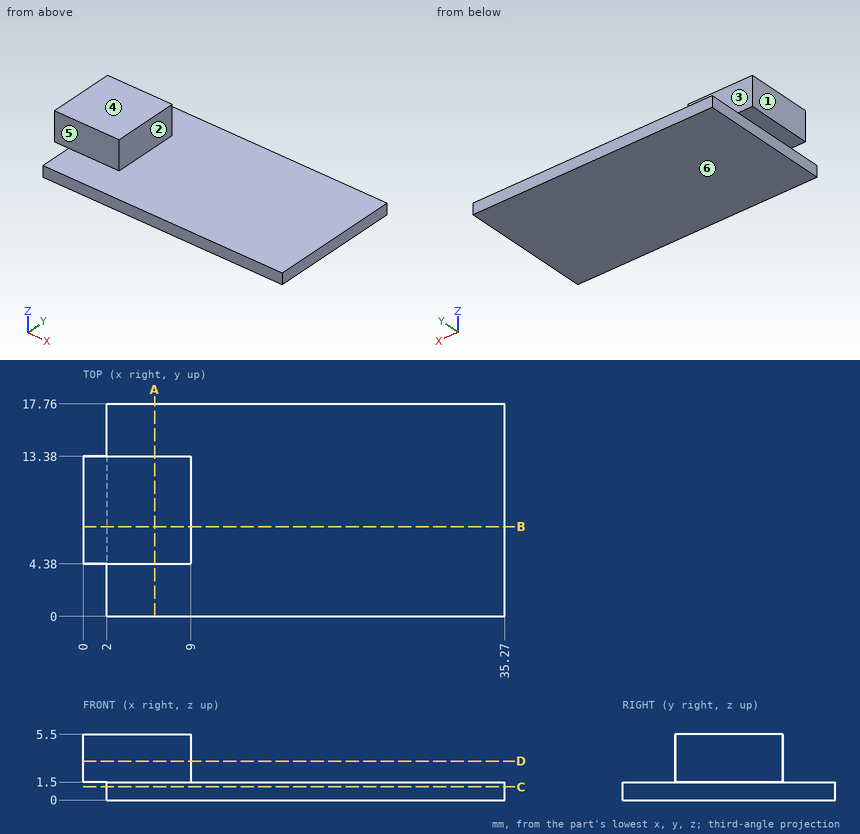
The figure shows three views and two pictorial views of one solid part (mm, origin at its lowest corner). Answer the questions. A direction names the side the tool comes from. Give positions to 0.01 mm unless a question says otherwise; leave off trailing zeros. Write each loop counter-clockwise with the first axis right and the second up, starting at its lowest first coordinate (ties: lowest second). Pieces come first, ordered by that corner, then holes. Notation, with made-up numbers: (32.25, 88.5) -> (56.25, 88.5) arc R34 ccw to (56.25, 118.5) -> close; hole circle Ø4 at (-30.75, 62). An arc over 180 degrees is marked (long way). Write each question's results on one line, items separated by ' | '.
1. Find section B-B on y = 7.5. Determine the outline of the cut face in (x, z).
Data:
outline: (0, 1.5) -> (2, 1.5) -> (2, 0) -> (35.27, 0) -> (35.27, 1.5) -> (9, 1.5) -> (9, 5.5) -> (0, 5.5) -> close
2. Find section C-C on z = 1.1. Determine the outline of the cut face in (x, y), and give its area (3 significant figures).
Data:
outline: (2, 0) -> (35.27, 0) -> (35.27, 17.76) -> (2, 17.76) -> close | area: 591 mm^2
3. Find section D-D on z = 3.25. Determine the outline of the cut face in (x, y), and give its area (3 significant figures).
Data:
outline: (0, 4.38) -> (9, 4.38) -> (9, 13.38) -> (0, 13.38) -> close | area: 81.0 mm^2
4. Each of these flat-tipped pins is pushed along its axis until it touches: pin 1 Ø3 at (x, y) = (27, 14.5) entering from +Z; pin 2 Ø3 at (y, z) = (10, 3.5) entering from +X; pin 3 Ø1.2 at (x, z) = (3.5, 4.5) entering from -Y. Where does it stop, or does it pass through?
Data:
pin 1: z = 1.5 | pin 2: x = 9 | pin 3: y = 4.38
5. A tool of negligible diameter and unlimited length cuts with its end or side. For the marked faces 1, 2 and 3, from which of +Z, -Z, +X, -X, +Y, -Y can it reach the whole face along a straight path? Write none if from no direction.
Data:
face 1: +Z, -Z, -X, +Y, -Y | face 2: +Z, +X, +Y, -Y | face 3: +Z, +X, -X, +Y
6. Straight lines are drawn through the part: L1, parallel to X at y = 13.25, z = 4.6; L2, parallel to X at y = 14.25, z = 0.4; L3, parallel to Z at x = 24.5, y = 11. For each, find the intervals that lie inside material, in ascending order.
Data:
L1: 0 to 9 | L2: 2 to 35.27 | L3: 0 to 1.5
7. Determine the mould class of the marked faces 4, 5 and 6 for opening direction Z: +Z half, -Z half, draft (parallel to the pull), parting line (faces both ways), or undercut.
Data:
face 4: +Z half | face 5: draft | face 6: -Z half
8. Find section A-A on x = 6. Determine the outline of the cut face in (y, z).
Data:
outline: (0, 0) -> (17.76, 0) -> (17.76, 1.5) -> (13.38, 1.5) -> (13.38, 5.5) -> (4.38, 5.5) -> (4.38, 1.5) -> (0, 1.5) -> close
